from build123d import *

# Parameters (mm, degrees)
F0_W          = 25.4
F0_H          = 25.4
F1_DEPTH      = 304.8
F1_DEPTH_BACK = 76.2
F2_R          = 6.35
F4_DEPTH      = 25.401


with BuildPart() as f1:
    # F0 (on Right) → F1 (new body, two sides)
    with BuildSketch(Plane.YZ) as f1_sk:
        Rectangle(F0_W, F0_H)
    extrude(amount=F1_DEPTH)
    extrude(f1_sk.sketch, amount=-F1_DEPTH_BACK)

    # F2
    f2_edges = [f1.edges().sort_by_distance(p)[0] for p in [
        (114.3, -12.7, 12.7),
        (114.3, 12.7, 12.7),
        (114.3, -12.7, -12.7),
        (114.3, 12.7, -12.7),
        (304.8, 12.7, 0),
        (304.8, 0, 12.7),
        (304.8, -12.7, 0),
        (304.8, 0, -12.7),
        (-76.2, 12.7, 0),
        (-76.2, 0, 12.7),
        (-76.2, -12.7, 0),
        (-76.2, 0, -12.7),
    ]]
    fillet(f2_edges, radius=F2_R)

    # F3 (on face) → F4 (cut, through all)
    with BuildSketch(Plane.XY.offset(12.7)):
        with BuildLine():
            ThreePointArc((114.2999998593, -6.35), (118.7901280108, -4.4901281103), (120.65, 0))
            ThreePointArc((120.65, 0), (118.7901280791, 4.4901280419), (114.3000000526, 6.35))
            ThreePointArc((114.3000000526, 6.35), (107.95, 9.66e-08), (114.2999998593, -6.35))
        make_face()
    extrude(amount=-F4_DEPTH, mode=Mode.SUBTRACT)


solid = f1.part
Input: part model. Units: mm. Frame: model coordinates. Give positions to 0.01 mm unless a question says otherwise; leave off trailing zeros. Order: outer loops, then holes, each group sorted by start corner. A loop starts at its lowest first (then second) coordinate and runs counter-clockwise, first axis right, second up. Notation, with made-up numbers: (59, 4.5) -> (96, 4.5) arc R5 cw to (96, 10.5) -> close; hole circle Ø1 at (-38, 71). An arc over 180 degrees is marked (long way). Use one line per item in the form item = value.
1) Section A-A, the plane x = 213. Return loops of the section in (y, z), and give its area (3 significant figures).
Response values:
outline = (-12.7, -6.35) arc R6.35 ccw to (-6.35, -12.7) -> (6.35, -12.7) arc R6.35 ccw to (12.7, -6.35) -> (12.7, 6.35) arc R6.35 ccw to (6.35, 12.7) -> (-6.35, 12.7) arc R6.35 ccw to (-12.7, 6.35) -> close
area = 611 mm^2
2) First-contact query: pin 1 Ø1.5 at (x, y) = (195, -7) entering from -Z; pin 2 Ø5 at (y, z) = (-10, -9) entering from -X; pin 3 Ø5 at (x, z) = (196, 10) entering from +Y (3 decimals). Flat tips, straight axial feed; report the tip coordinate or a pass-through.
Response values:
pin_1 = -12.7
pin_2 = -75.87
pin_3 = 12.595
3) Line query: probe 1 along X at (y, z) = (4.25, -9.75); probe 2 along X at (y, z) = (-2.75, 10.5); probe 3 along X at (y, z) = (6.75, -4.25). Output: solid intervals per line, ascending.
Response values:
probe_1 = -75.21 to 109.58, 119.02 to 303.81
probe_2 = -74.66 to 108.58, 120.02 to 303.26
probe_3 = -76.19 to 304.79
